Geometry check sheet. Reference: the model listing, model coordinates, mm. A direction names the side the tool comes from. Give positions to 0.01 mm unless a question says otherwise; leave off trailing zeros. Loops run counter-clockwise (first coordinate to the right, second up) from the corner with the lowest first, then second, coordinate; pieces in that order, holes last. Notation, with made-up numbers: (53.25, 6) -> (64.25, 6) arc R18 ccw to (64.25, 25) -> close; hole circle Ø8 at (-24, 34). An arc over 180 degrees is marked (long way). Answer as a JSON object with one key per item and string values.
from build123d import *

# Parameters (mm, degrees)
FILLET1_R   = 0.25
HEX_2_DEPTH = 2.08


with BuildPart() as part:
    # BodySke → BaseBody (revolve)
    with BuildSketch(Plane.XY):
        with BuildLine():
            Line((28.3, 0), (28.3, 2.4455))
            Line((28.3, 2.4455), (27.7455, 3))
            Line((27.7455, 3), (3.3, 3))
            Line((3.3, 3), (3.3, 5.25))
            Line((3.3, 5.25), (2.92, 5.25))
            ThreePointArc((2.92, 5.25), (1.224500646, 4.199464996), (0, 2.625))
            Line((0, 2.625), (0, 0))
            Line((0, 0), (28.3, 0))
        make_face()
    revolve(axis=Axis((0, 0, 0), (1, 0, 0)))

    # Fillet1
    fillet1_edges = [part.edges().sort_by_distance(p)[0] for p in [
        (3.3, -3, 0),
    ]]
    fillet(fillet1_edges, radius=FILLET1_R)

    # Sketch2 → PreBroach (revolve, cut)
    with BuildSketch(Plane.XY):
        Polygon((0, 2), (2.08, 2), (3.234700538, 0), (0, 0), align=None)
    revolve(axis=Axis((0, 0, 0), (1, 0, 0)), mode=Mode.SUBTRACT)

    # Sketch3 → Hex 2 (cut)
    with BuildSketch(Plane(origin=(0, 0, 0), x_dir=(0, 0, -1), z_dir=(1, 0, 0))):
        Polygon((-2, -1.154700538), (-2, 1.154700538), (0, 2.309401077), (2, 1.154700538), (2, -1.154700538), (0, -2.309401077), align=None)
    extrude(amount=HEX_2_DEPTH, mode=Mode.SUBTRACT)


solid = part.part
1) Section check A-A on x = 24.25. Record the cut outline in (y, z).
Geometry check:
{"outline": "circle Ø6 at (0, 0)"}
2) Draft check along Z on faces 1 (the face through (15, -3, 0)), 2 (the face through (3.3, 0.1, -3.4)), 3 (the face through (1.025, -1.724, -1.014)). Enter one of: pulls with the +Z half, pulls with the -Z half, needs draft (parallel to the pull), parting line crosses it, or undercut.
Geometry check:
{"face 1": "parting line crosses it", "face 2": "needs draft", "face 3": "undercut"}
3) Material ranges on line 1 along Z through (x, y) = (10.75, 0.25); line 2 along Z through (x, y) = (8.25, 2.5); line 3 along X through (y, z) = (-0.75, -3), recorded low to high. Write a range as from..to.
Geometry check:
{"line 1": "z = -2.99..2.99", "line 2": "z = -1.66..1.66", "line 3": "x = 0.27..3.36"}
4) Section check B-B on z = -4. Record the cut outline in (x, y), plus the area to 3 significant figures.
Geometry check:
{"outline": "(2.92, -3.4) -> (3.3, -3.4) -> (3.3, 3.4) -> (2.92, 3.4) arc R3.99 ccw to start", "area": "11.7 mm2"}
5) Tool access check on faces 4 (the face through (1.03, 1.74, -0.99)), 5 (the face through (3.1, 5, 1.6)). Record the directions out of +Z, -Z, +X, -X, +Y, -Y that give a thin tool (end or side, any length) a straight path to the whole face; none if there is none.
Geometry check:
{"face 4": "-X", "face 5": "+X, -X"}
6) Depth check by flat-ended pin: P1, Ø4, axis at y = 0.5, z = 0.5, coming from the -X side; P2, Ø5, axis at x = 12.5, y = -0.5, coming from the +Z side; P3, Ø6, axis at x = 17, z = 3, coming from the +Y side; P4, Ø1, axis at x = 8, y = 1.5, coming from the +Z side. Enter the tip coordinate at first touch or a pass-through.
Geometry check:
{"P1": "stops at x = 0", "P2": "stops at z = 3", "P3": "stops at y = 3", "P4": "stops at z = 2.83"}
